Here's the drawing with two shaded views (mm, measured from the low corner). I have some questions. A direction names the side the tool comes from. Give positions to 0.01 mm unless a question says otherwise; leave off trailing zeros. Write each loop counter-clockwise with the first axis right and the second up, starting at its lowest first coordinate (ties: lowest second). Pieces come first, ordered by that corner, then holes. Notation, with made-up numbers: M 60.5,-10.5 L 67.5,-10.5 A12 cw 67.5,4.5 Z; hole C 30.25,49.25 d5. An arc over 180 degrees is marked long. Use one line per item in the form item = value. Start each with the question number.
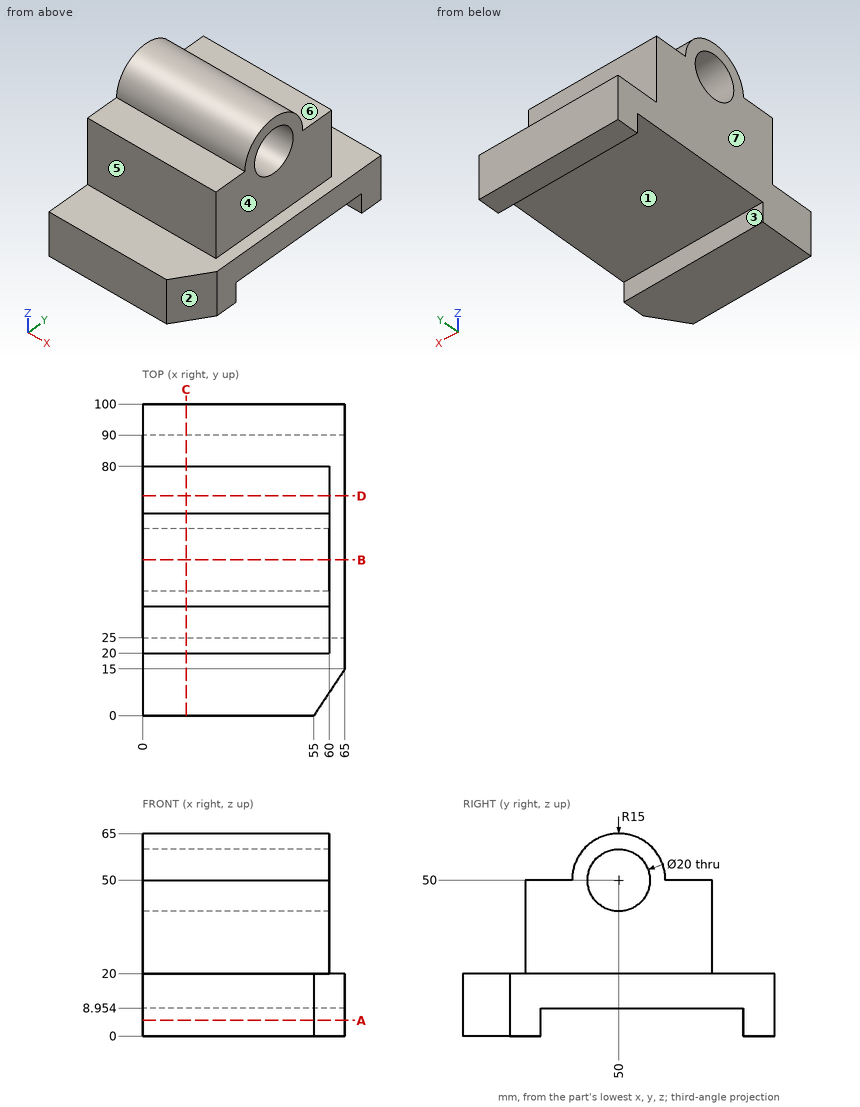
1) Will these pins go through, and if not, where does the flat tip stop? P1, Ø8, axis at x = 22, z = 46, coming from the -Y side; P2, Ø2, axis at x = 20, y = 49.5, coming from the +Z side; P3, Ø12, axis at x = 47.5, y = 22.5, coming from the +Z side; P4, Ø9, axis at x = 23, z = 39, coming from the +Y side.
2) Suppose I cut it at B-B, the plane y = 50. List the corners of the cut face in (x, z) for me, and give its area (3 significant figures).
3) On a 3-axis mill with a long thin cutter (end or side, diameter ignored), from which of +Z, -Z, +X, -X, +Y, -Y can I reach the whole of each face in a straight line? I mean the marked faces 5, 6 and 7. Say none if no direction works.
4) Thinking about a two-plate mould opening in Y: for the marked faces 1, 2, 3 and 4, which applies, released by +Y, released by -Y, zero draft, split by the parting line, or undercut?
5) Suppose I cut it at D-D, the plane y = 70.5. List the corners of the cut face in (x, z) for me, and give its area (3 significant figures).
6) Suppose I cut it at A-A, the plane z = 5. List the corners of the cut face in (x, y) for me.
7) Please list where these lines run through material, in increasing order: line 1 (Z direction, x = 12, y = 50); line 2 (X direction, y = 53, z = 37); line 3 (Y direction, x = 56.5, z = 28.5).
8) Suppose I cut it at C-C, the plane x = 14. List the corners of the cut face in (y, z) for me, and give its area (3 significant figures).
Checks:
q1.P1 = 20
q1.P2 = 65
q1.P3 = 50
q1.P4 = 80
q2.outline = M 0,8.95 L 65,8.95 L 65,20 L 60,20 L 60,40 L 0,40 Z; M 0,60 L 60,60 L 60,65 L 0,65 Z
q2.area = 2,220 mm^2
q3.face_5 = +Z, +X, -X, -Y
q3.face_6 = +Z, +X, -X, +Y
q3.face_7 = +Z, -Z, -X, +Y, -Y
q4.face_1 = undercut
q4.face_2 = released by -Y
q4.face_3 = undercut
q4.face_4 = zero draft
q5.outline = M 0,8.95 L 65,8.95 L 65,20 L 60,20 L 60,50 L 0,50 Z
q5.area = 2,520 mm^2
q6.outline = M 0,0 L 55,0 L 65,15 L 65,25 L 0,25 Z; M 0,90 L 65,90 L 65,100 L 0,100 Z
q7.line_1 = 8.95 to 40, 60 to 65
q7.line_2 = 0 to 60
q7.line_3 = 20 to 80
q8.outline = M 0,0 L 25,0 L 25,8.95 L 90,8.95 L 90,0 L 100,0 L 100,20 L 80,20 L 80,50 L 65,50 A15 ccw 35,50 L 20,50 L 20,20 L 0,20 Z; hole C 50,50 d20
q8.area = 3,260 mm^2
